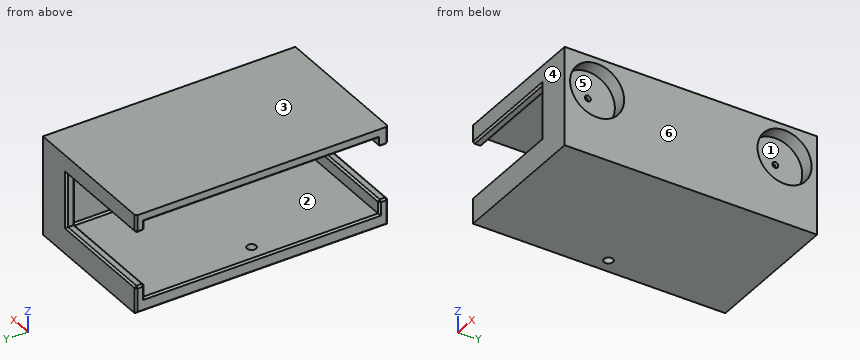
```python
from build123d import *

# Parameters (mm, degrees)
F1_DEPTH  = 130
F2_DEPTH  = 5
F4_DEPTH  = 5
F5_SIZE   = 1
F7_DEPTH  = 8
F8_DEPTH  = 20
F10_DEPTH = 10


with BuildPart() as f1:
    # F0 (on Front) → F1 (new body)
    with BuildSketch(Plane.XZ):
        Polygon((0, -55), (0, 0), (-80, 0), (-80, -5), (-10, -5), (-10, -47.5), (-80, -47.5), (-80, -55), align=None)
    extrude(amount=F1_DEPTH)

    # F0 (on Front) + F1_face (on face) → F2 (join)
    with BuildSketch(Plane.XZ):
        Polygon((0, -55), (0, 0), (-80, 0), (-80, -5), (-10, -5), (-10, -47.5), (-80, -47.5), (-80, -55), align=None)
        Polygon((-10, -5), (-80, -5), (-80, -10), (-20, -10), (-20, -40), (-80, -40), (-80, -47.5), (-10, -47.5), align=None)
    with BuildSketch(Plane(origin=(-29.5614035088, 0, -30.1096491228), x_dir=(1, 0, 0), z_dir=(0, 1, 0))):
        Polygon((29.5614035088, -30.1096491228), (29.5614035088, 24.8903508772), (-50.4385964912, 24.8903508772), (-50.4385964912, 17.3903508772), (19.5614035088, 17.3903508772), (19.5614035088, -25.1096491228), (-50.4385964912, -25.1096491228), (-50.4385964912, -30.1096491228), align=None)
    extrude(amount=-F2_DEPTH, dir=(0, -1, 0))

    # F3 (on face) → F4 (join)
    with BuildSketch(Plane.XZ.offset(130)):
        Polygon((-10, -5), (-80, -5), (-80, -10), (-20, -10), (-20, -40), (-80, -40), (-80, -47.5), (-10, -47.5), align=None)
        Polygon((-80, 0), (-80, -5), (-10, -5), (-10, -47.5), (-80, -47.5), (-80, -55), (0, -55), (0, 0), align=None)
    extrude(amount=F4_DEPTH)

    # F5
    f5_edges = [f1.edges().sort_by_distance(p)[0] for p in [
        (-50, -135, -40),
        (-20, -135, -25),
        (-50, -135, -10),
        (-50, -130, -40),
        (-20, -130, -25),
        (-50, -130, -10),
        (-50, 0, -10),
        (-50, 5, -10),
        (-20, 0, -25),
        (-20, 5, -25),
        (-50, 5, -40),
        (-80, 2.5, -40),
        (-50, 0, -40),
        (-80, 2.5, -10),
        (-80, -130, -43.75),
        (-10, -65, -47.5),
        (-80, -65, -5),
        (-80, 0, -7.5),
        (-80, -65, -47.5),
        (-80, 0, -43.75),
        (-80, 5, -47.5),
        (-80, -132.5, -40),
        (-80, -135, -47.5),
        (-80, -65, -55),
        (-80, -132.5, -10),
        (-80, 5, -5),
        (-80, -135, -5),
    ]]
    chamfer(f5_edges, length=F5_SIZE)

    # F6 (on face) → F7 (cut)
    with BuildSketch(Plane.YZ):
        with BuildLine():
            ThreePointArc((-118.65, -18), (-117, -16.35), (-115.35, -18))
            Line((-115.35, -18), (-102, -18))
            ThreePointArc((-102, -18), (-117, -3), (-132, -18))
            Line((-132, -18), (-118.65, -18))
        make_face()
        with BuildLine():
            Line((-102, -18), (-115.35, -18))
            ThreePointArc((-115.35, -18), (-117, -19.65), (-118.65, -18))
            Line((-118.65, -18), (-132, -18))
            ThreePointArc((-132, -18), (-117, -33), (-102, -18))
        make_face()
        with BuildLine():
            ThreePointArc((2, -18), (-13, -3), (-28, -18))
            Line((-28, -18), (-14.65, -18))
            ThreePointArc((-14.65, -18), (-13, -16.35), (-11.35, -18))
            Line((-11.35, -18), (2, -18))
        make_face()
        with BuildLine():
            Line((-14.65, -18), (-28, -18))
            ThreePointArc((-28, -18), (-13, -33), (2, -18))
            Line((2, -18), (-11.35, -18))
            ThreePointArc((-11.35, -18), (-13, -19.65), (-14.65, -18))
        make_face()
    extrude(amount=-F7_DEPTH, mode=Mode.SUBTRACT)

    # F8 (cut): faces of the model
    f8_faces = [f1.faces().sort_by_distance(p)[0] for p in [
        (0, -13, -18),
        (0, -117, -18),
    ]]
    extrude(f8_faces, amount=-F8_DEPTH, mode=Mode.SUBTRACT)

    # F9 (on face) → F10 (cut)
    with BuildSketch(Plane(origin=(0, 0, -55), x_dir=(1, 0, 0), z_dir=(0, 0, -1))):
        with BuildLine():
            ThreePointArc((-73.5, 65), (-71, 62.5), (-68.5, 65))
            ThreePointArc((-68.5, 65), (-71, 67.5), (-73.5, 65))
        make_face()
    extrude(amount=-F10_DEPTH, mode=Mode.SUBTRACT)


solid = f1.part
```
Read the model definition and answer for the solid it produces. Units are mm, in the model's axes. Face numbers are marked on the shaded views. A direction names the side the tool comes from. Round coordinates to 2 decimals unless told otherwise and drop trailing zeros. Write each loop counter-clockwise with the first axis right and the second up, starting at its lowest first coordinate (ties: lowest second). Pieces come first, ordered by that corner, then holes. Notation, with made-up numbers: (66.25, 27) - (93.25, 27) arc R14 ccw to (93.25, 51) - close; hole circle Ø6 at (34, -26). An arc over 180 degrees is marked (long way). One line per item, written item: value.
Q1. Which of the six approach directions +Z, -Z, +X, -X, +Y, -Y give full straight-line access (tool end or side, diameter ignored) to the marked faces 1, 2 and 3?
The answers:
face 1: +X
face 2: -X
face 3: +Z, +X, -X, +Y, -Y
Q2. Straight lines are drawn through the part: line 1 (Y direction, x = -3, z = -18); line 2 (X direction, y = -65, z = -50.25); line 3 (Z direction, x = -2, y = -117). For each, find the intervals that lie inside material, in ascending order. Write a range as from..to.
The answers:
line 1: y = -135..-132, -102..-28, 2..5
line 2: x = -80..-73.5, -68.5..0
line 3: z = -55..-33, -3..0
Q3. Find section A-A (y = -65). Determine the outline of the cut face in (x, z).
The answers:
outline: (-80, -54) - (-79, -55) - (-73.5, -55) - (-73.5, -47.5) - (-79, -47.5) - (-80, -48.5) - close; (-80, -4) - (-79, -5) - (-10, -5) - (-10, -46.5) - (-11, -47.5) - (-68.5, -47.5) - (-68.5, -55) - (0, -55) - (0, 0) - (-80, 0) - close
Q4. Find section D-D (x = -71). Determine the outline of the cut face in (y, z).
The answers:
outline: (-135, -55) - (-67.5, -55) - (-67.5, -47.5) - (-130, -47.5) - (-130, -41) - (-131, -40) - (-134, -40) - (-135, -41) - close; (-135, -9) - (-134, -10) - (-131, -10) - (-130, -9) - (-130, -5) - (0, -5) - (0, -9) - (1, -10) - (4, -10) - (5, -9) - (5, 0) - (-135, 0) - close; (-62.5, -55) - (5, -55) - (5, -41) - (4, -40) - (1, -40) - (0, -41) - (0, -47.5) - (-62.5, -47.5) - close
Q5. Find section B-B (x = -52). Determine the outline of the cut face in (y, z), and give its area (3 significant figures).
The answers:
outline: (-135, -55) - (5, -55) - (5, -41) - (4, -40) - (1, -40) - (0, -41) - (0, -47.5) - (-130, -47.5) - (-130, -41) - (-131, -40) - (-134, -40) - (-135, -41) - close; (-135, -9) - (-134, -10) - (-131, -10) - (-130, -9) - (-130, -5) - (0, -5) - (0, -9) - (1, -10) - (4, -10) - (5, -9) - (5, 0) - (-135, 0) - close
area: 1,870 mm2
Q6. Find section C-C (z = -18). Determine the outline of the cut face in (x, y).
The answers:
outline: (-20, -134) - (-19, -135) - (0, -135) - (0, -132) - (-8, -132) - (-8, -118.65) - (-10, -118.65) - (-10, -130) - (-19, -130) - (-20, -131) - close; (-20, 1) - (-19, 0) - (-10, 0) - (-10, -11.35) - (-8, -11.35) - (-8, 2) - (0, 2) - (0, 5) - (-19, 5) - (-20, 4) - close; (-10, -115.35) - (-8, -115.35) - (-8, -102) - (0, -102) - (0, -28) - (-8, -28) - (-8, -14.65) - (-10, -14.65) - close
Q7. Each of these flat-tipped pins is pushed along its axis until it touches: P1, Ø9, axis at y = -12, z = -15.5, coming from the +X side; P2, Ø5.5, axis at y = -13, z = -18, coming from the -X side; P3, Ø3.5, axis at y = 3, z = -24.5, coming from the -X side. Where does it stop, or does it pass through?
The answers:
P1: stops at x = -8
P2: stops at x = -10
P3: stops at x = -20
Q8. For a pull along Y with two mould halves and no side action, classify the marked faces 4, 5 and 6 as pulls with the +Y half, pulls with the -Y half, needs draft (parallel to the pull), parting line crosses it, or undercut.
The answers:
face 4: pulls with the -Y half
face 5: undercut
face 6: needs draft
